```python
from build123d import *

# Parameters (mm, degrees)
SKETCH1_W                                      = 17
SKETCH1_H                                      = 31
BOSS_EXTRUDE1_DEPTH                            = 4.5
SKETCH2_R                                      = 4
SKETCH2_R_2                                    = 1.5
BOSS_EXTRUDE2_DEPTH                            = 7.75
FILLET2_R                                      = 15
CSK_FOR_M5_FLAT_HEAD_MACHINE_SCREW1_AT_2_COUNT = 2
CSK_FOR_M5_FLAT_HEAD_MACHINE_SCREW1_AT_2_PITCH = 14.5
BOSS_EXTRUDE4_DEPTH                            = 7.75
LPATTERN1_START                                = 15.5
LPATTERN1_OUTLINE_R                            = 1.5
LPATTERN1_DEPTH                                = 7.75
SKETCH7_W                                      = 1
SKETCH7_H                                      = 7.75
CUT_EXTRUDE1_DEPTH                             = 36.640566774


# Read off the part's stored shape, not the designer's step: LPattern1
with BuildPart() as part:
    # Sketch1 → Boss-Extrude1 (new body)
    with BuildSketch(Plane.XY):
        with Locations((-8.5, 15.5)):
            Rectangle(SKETCH1_W, SKETCH1_H)
    extrude(amount=BOSS_EXTRUDE1_DEPTH)

    # Sketch2 → Boss-Extrude2 (add)
    with BuildSketch(Plane(origin=(0, 0, 0), x_dir=(1, 0, 0), z_dir=(0, 1, 0))):
        with Locations((3, -4.5)):
            Circle(SKETCH2_R)
        with Locations(Location((3, -4.5, 0), (0, 0, 270))):
            Circle(SKETCH2_R_2, mode=Mode.SUBTRACT)
    extrude(amount=BOSS_EXTRUDE2_DEPTH)

    # Fillet2
    # the kernel refuses this fillet: 15 mm, written as the material it adds along each edge
    with BuildSketch(Plane(origin=(0, 7.75, 1.854248689), x_dir=(0.9211814219318991, 0, -0.389133380587588), z_dir=(0, -1, 0))) as fillet2_piece_1:
        with BuildLine():
            CenterArc((9.970466155, -13.517314112), FILLET2_R, 115.689791336, 12.37807292)
            Line((0.721550061, -1.708099444), (0.536571739, -1.471915151))
            ThreePointArc((0.536571739, -1.471915151), (0.084420604, -0.970789736), (-0.276354427, -0.116740014))
            Line((-0.276354427, -0.116740014), (0.130049559, 0.270346282))
            ThreePointArc((0.130049559, 0.270346282), (1.733994114, -0.095382903), (3.337938669, 0.270346282))
            Line((3.337938669, 0.270346282), (3.467988228, 0))
        make_face()
    extrude(amount=7.75)

    # Sketch4 → CSK for M5 Flat Head Machine Screw1 (revolve, cut)
    with BuildSketch(Plane(origin=(-7.5, 8.25, 4.5), x_dir=(0, -1, 0), z_dir=(1, 0, 0))):
        Polygon((0, 0), (0, 4.5), (2.75, 4.5), (2.75, 2.45), (5.2, 0), align=None)
    csk_for_m5_flat_head_machine_screw1 = revolve(axis=Axis((-7.5, 8.25, 10.85), (0, 0, -1)), mode=Mode.SUBTRACT)

    # CSK for M5 Flat Head Machine Screw1 at 2: CSK for M5 Flat Head Machine Screw1 ×2
    with Locations(*[(0, i * CSK_FOR_M5_FLAT_HEAD_MACHINE_SCREW1_AT_2_PITCH, 0) for i in range(1, CSK_FOR_M5_FLAT_HEAD_MACHINE_SCREW1_AT_2_COUNT)]):
        add(csk_for_m5_flat_head_machine_screw1, mode=Mode.SUBTRACT)

    # Sketch6 → Boss-Extrude4 (add)
    with BuildSketch(Plane.XZ):
        Polygon((0, 0), (6.999251024, 0), (6.999251024, 4.577403122), align=None)
    extrude(amount=-BOSS_EXTRUDE4_DEPTH)

    # LPattern1 outline → LPattern1 (add)
    with BuildSketch(Plane(origin=(0, 0, 0), x_dir=(1, 0, 0), z_dir=(0, 1, 0)).offset(LPATTERN1_START)):
        with BuildLine():
            Line((6.999251024, 0), (0, 0))
            Line((0, 0), (0, -4.5))
            Line((0, -4.5), (-1, -4.5))
            ThreePointArc((-1, -4.5), (3.038703373, -8.499812752), (6.999251024, -4.422596878))
            Line((6.999251024, -4.422596878), (6.999251024, 0))
        make_face()
        with Locations((3, -4.5)):
            Circle(LPATTERN1_OUTLINE_R, mode=Mode.SUBTRACT)
    extrude(amount=LPATTERN1_DEPTH)

    # Sketch7 → Cut-Extrude1 (cut, through all)
    with BuildSketch(Plane.XY.offset(4.5)):
        with Locations((-0.5, 11.625)):
            Rectangle(SKETCH7_W, SKETCH7_H)
        with Locations((-0.5, 27.125)):
            Rectangle(SKETCH7_W, SKETCH7_H)
    extrude(amount=-CUT_EXTRUDE1_DEPTH, mode=Mode.SUBTRACT)


solid = part.part
```
Geometry check sheet. Reference: the model listing, model coordinates, mm. A direction names the side the tool comes from. Round coordinates to 2 decimals unless told otherwise and drop trailing zeros. Loops run counter-clockwise (first coordinate to the right, second up) from the corner with the lowest first, then second, coordinate; pieces in that order, holes last. Notation, with made-up numbers: (69, 45.25) - (120, 45.25) arc R25 ccw to (120, 65.25) - close; hole circle Ø6 at (19, -2.5). An arc over 180 degrees is marked (long way). Use a Markdown table: item, result.
Q1. Cross-section at D-D on y = 8.25. Record the cut outline in (x, z), plus the area to 3 significant figures.
Solutions:
| item | result |
|---|---|
| outline | (-17, 0) - (-10.25, 0) - (-10.25, 2.05) - (-12.7, 4.5) - (-17, 4.5) - close; (-4.75, 0) - (-1, 0) - (-1, 4.5) - (-2.3, 4.5) - (-4.75, 2.05) - close |
| area | 41.2 mm2 |
Q2. Cross-section at C-C on x = 3. Record the cut outline in (y, z), plus the area to 4 significant figures.
Solutions:
| item | result |
|---|---|
| outline | (0, 0) - (7.75, 0) - (7.75, 3) - (0, 3) - close; (0, 6) - (7.75, 6) - (7.75, 8.5) - (0, 8.5) - close; (15.5, 0) - (23.25, 0) - (23.25, 3) - (15.5, 3) - close; (15.5, 6) - (23.25, 6) - (23.25, 8.5) - (15.5, 8.5) - close |
| area | 85.25 mm2 |
Q3. Material ranges on line 1 (Y direction, x = -7.5, z = 1.25); line 2 (X direction, y = 8.25, z = 1.4); line 3 (X direction, y = 22.75, z = 1.05), recorded low to high.
Solutions:
| item | result |
|---|---|
| line 1 | y = 0 to 5.5, 11 to 20, 25.5 to 31 |
| line 2 | x = -17 to -10.25, -4.75 to -1 |
| line 3 | x = -17 to -10.25, -4.75 to 7 |
Q4. Go/stop test with flat-tipped pins: P1, Ø5, axis at x = 3, z = 4.5, coming from the +Y side; P2, Ø2, axis at x = -12.5, y = 11.5, coming from the +Z side; P3, Ø4.5, axis at x = -7.5, y = 22.75, coming from the +Z side; P4, Ø5, axis at x = -6, y = 10, coming from the +Z side. Record where each tip stops, or that it passes through.
Solutions:
| item | result |
|---|---|
| P1 | stops at y = 23.25 |
| P2 | stops at z = 4.5 |
| P3 | passes through |
| P4 | stops at z = 4.1 |
Q5. Access from +Z, -Z, +X, -X, +Y, -Y to the whole of each face (thin tool, end or side, straight path). Record for faces 4 (the flat face through (3, 15.5, 2)), 5 (the flat face through (4, 23.25, 3)), 6 (the cylindrical face through (-7.6, 25.5, 1)).
Solutions:
| item | result |
|---|---|
| face 4 | +Z, -Z, +X |
| face 5 | +Z, -Z, +X, +Y |
| face 6 | +Z, -Z |
Q6. Draft check along Y on faces 1 (the flat face through (-5, 0, 3)), 2 (the flat face through (3, 7.75, 2)), 3 (the flat face through (-9, 16, 4.5)). Enter one of: released by +Y, released by -Y, zero draft, split by the parting line, or undercut.
Solutions:
| item | result |
|---|---|
| face 1 | released by -Y |
| face 2 | undercut |
| face 3 | zero draft |
Q7. Cross-section at A-A on x = -7.5. Record the cut outline in (y, z).
Solutions:
| item | result |
|---|---|
| outline | (0, 0) - (5.5, 0) - (5.5, 2.05) - (3.05, 4.5) - (0, 4.5) - close; (11, 0) - (20, 0) - (20, 2.05) - (17.55, 4.5) - (13.45, 4.5) - (11, 2.05) - close; (25.5, 0) - (31, 0) - (31, 4.5) - (27.95, 4.5) - (25.5, 2.05) - close |
Q8. Cross-section at B-B on y = 22.75. Record the cut outline in (x, z), plus the area to 3 significant figures.
Solutions:
| item | result |
|---|---|
| outline | (-17, 0) - (-10.25, 0) - (-10.25, 2.05) - (-12.7, 4.5) - (-17, 4.5) - close; (-4.75, 0) - (7, 0) - (7, 4.42) arc R4 ccw (long way) to (-1, 4.5) - (-2.3, 4.5) - (-4.75, 2.05) - close; hole circle Ø3 at (3, 4.5) |
| area | 95.3 mm2 |
